The model under review builds one solid part; all positions refer to its coordinate system, in mm. A direction names the side the tool comes from. Coordinates: 2 decimals unless noted, no trailing zeros. Write each loop counter-clockwise with the first axis right and the second up, starting at its lowest first coordinate (ties: lowest second). Pieces come first, ordered by that corner, then holes. Notation, with made-up numbers: (69.25, 1.5) -> (105.25, 1.5) arc R17 cw to (105.25, 33.5) -> close; hole circle Ø2 at (67.25, 86.5). An arc over 180 degrees is marked (long way). Put each result on its own line as item: value. Start each with the question number.
from build123d import *

# Parameters (mm, degrees)
BOX001_W          = 10
BOX001_H          = 20
BOX001_DEPTH      = 10
CYLINDER001_R     = 10
CYLINDER001_DEPTH = 40
CYLINDER002_R     = 12
CYLINDER002_DEPTH = 40


with BuildPart() as cubo:
    # Box001 → Box001 (new body)
    with BuildSketch(Plane(origin=(0, -20, 0), x_dir=(1, 0, 0), z_dir=(0, 0, 1))):
        with Locations((5, 10)):
            Rectangle(BOX001_W, BOX001_H)
    extrude(amount=BOX001_DEPTH)


with BuildPart() as cilindro:
    # Cylinder001 → Cylinder001 (new body)
    with BuildSketch(Plane.XY):
        Circle(CYLINDER001_R)
    extrude(amount=CYLINDER001_DEPTH)


with BuildPart() as exterior_torre:
    # Cylinder002 → Cylinder002 (new body)
    with BuildSketch(Plane.XY):
        Circle(CYLINDER002_R)
    extrude(amount=CYLINDER002_DEPTH)

    # Cut: cut Cilindro
    add(cilindro.part, mode=Mode.SUBTRACT)

    # Cut001: cut Cubo
    add(cubo.part, mode=Mode.SUBTRACT)


solid = exterior_torre.part
1. Wall thickness on line 1 (Y direction, x = 0.25, z = 31.5); line 2 (X direction, y = 2, z = 31.5): over which ranges is each line inside the solid? List them lowest first. Write a range as from..to.
2. Consider section C-C on z = 37. State the section outline as (x, y) points.
3. Insertion check: P1, Ø7.5, axis at y = -2.5, z = 6, coming from the -X side; P2, Ø8, axis at x = -9.5, z = 32, coming from the +Y side; P3, Ø10, axis at y = -7, z = 10, coming from the -X side; P4, Ø2, axis at y = -10.5, z = 6.5, coming from the +X side. Each pin has a flat end and moves straight along its axis. Give the tip position at first contact, or say it passes through.
4. Consider section D-D on x = -6.5. State the section outline as (y, z) points.
5. Consider section A-A on x = -4. State the section outline as (y, z) points.
6. Consider section B-B on y = -5. State the section outline as (x, z) points, then the cut area to 3 significant figures.
7. Tool access review of faces 5 (the flat face through (6, -9, 10)), 6 (the cylindrical face through (-7.37, 6.76, 19.72)): name each direction out of +Z, -Z, +X, -X, +Y, -Y from which nothing blocks a thin tool from reaching the whole face with its end or side.
8. The part is to be moulded in two halves that separate along X. For faces 1 (the flat face through (0, -11, 5)), 2 (the flat face through (10, -3, 5)), 3 (the cylindrical face through (-8.844, 8.11, 19.72)), 4 (the flat face through (-6.3, 8.1, 0)), say which applies: released by +X, released by -X, zero draft, split by the parting line, or undercut.
Output values:
1. line 1: y = -12..-10, 10..12
1. line 2: x = -11.83..-9.8, 9.8..11.83
2. outline: circle Ø24 at (0, 0); hole circle Ø20 at (0, 0)
3. P1: stops at x = -12
3. P2: stops at y = 10.67
3. P3: stops at x = -11.83
3. P4: stops at x = 0
4. outline: (-10.09, 0) -> (-7.6, 0) -> (-7.6, 40) -> (-10.09, 40) -> close; (7.6, 0) -> (10.09, 0) -> (10.09, 40) -> (7.6, 40) -> close
5. outline: (-11.31, 0) -> (-9.17, 0) -> (-9.17, 40) -> (-11.31, 40) -> close; (9.17, 0) -> (11.31, 0) -> (11.31, 40) -> (9.17, 40) -> close
6. outline: (-10.91, 0) -> (-8.66, 0) -> (-8.66, 40) -> (-10.91, 40) -> close; (8.66, 10) -> (10, 10) -> (10, 0) -> (10.91, 0) -> (10.91, 40) -> (8.66, 40) -> close
6. area: 166 mm^2
7. face 5: -Z, -Y
7. face 6: +Z, -Z
8. face 1: released by +X
8. face 2: undercut
8. face 3: split by the parting line
8. face 4: zero draft
